The model under review builds one solid part; all positions refer to its coordinate system, in mm. A direction names the side the tool comes from. Give positions to 0.01 mm unless a question says otherwise; leave off trailing zeros. Loops run counter-clockwise (first coordinate to the right, second up) from the corner with the lowest first, then second, coordinate; pieces in that order, holes last. Notation, with made-up numbers: (-36, -13.5) -> (-16, -13.5) arc R17 cw to (-16, 1.5) -> close; hole circle Ø10 at (26, 74.5). An arc over 180 degrees is marked (long way). Write each question's results on one line, items separated by ' | '. Start each with the question number.
Q1. Mouldability with a two-part tool opening along Y and no side actions: class faces 1 (the face through (197, 4, 0)), 2 (the face through (197, 0, 19)), 3 (the face through (390, -4.5, 2.7)) as released by +Y, released by -Y, zero draft, split by the parting line, or undercut.
Q2. We need section C-C (z = -1.5). Write out the cut boundary in (x, y).
Q3. We need section B-B (x = 272). Write out the cut boundary in (y, z).
Q4. Machinability: for faces 4 (the face through (197, 0, -17.5)), 5 (the face through (197, 0, -19)), which of the approach directions +Z, -Z, +X, -X, +Y, -Y give a long, thin tool a straight path to every point of the face, cutting with its end or side? Answer none if there is none.
Q5. We need section A-A (y = 0.5). Write out the cut boundary in (x, z).
Q6. Wall thickness on L1, parallel to Z at x = 326, y = -2.25; L2, parallel to Y at x = 21, z = -13; L3, parallel to X at y = 4.5, z = 8.5: over which ranges is each line inside the solid? List them lowest first. Write a range as [from, to].
from build123d import *

# Parameters (mm, degrees)
SKETCH1_W               = 38
SKETCH1_H               = 11
SKETCH1_W_2             = 35
SKETCH1_H_2             = 8
BOSS_EXTRUDE1_DEPTH     = 400
CUT_EXTRUDE1_DEPTH      = 1
CUT_EXTRUDE1_DEPTH_BACK = 39
CUT_EXTRUDE3_DEPTH      = 1
CUT_EXTRUDE3_DEPTH_BACK = 39


with BuildPart() as part:
    # Sketch1 → Boss-Extrude1 (new body)
    with BuildSketch(Plane(origin=(0, 0, 0), x_dir=(0, 0, -1), z_dir=(1, 0, 0))):
        Rectangle(SKETCH1_W, SKETCH1_H)
        Rectangle(SKETCH1_W_2, SKETCH1_H_2, mode=Mode.SUBTRACT)
    extrude(amount=BOSS_EXTRUDE1_DEPTH)

    # Sketch2 → Cut-Extrude1 (cut, two sides)
    with BuildSketch(Plane(origin=(0, 0, -19), x_dir=(-1, 0, 0), z_dir=(0, 0, -1))) as cut_extrude1_sk:
        Polygon((572.970352137, 578.470352137), (0, 5.5), (-11, -5.5), (-583.970352137, -578.470352137), (561.970352137, -1724.411056412), (1718.911056412, -567.470352137), align=None)
    extrude(amount=CUT_EXTRUDE1_DEPTH, mode=Mode.SUBTRACT)
    extrude(cut_extrude1_sk.sketch, amount=-CUT_EXTRUDE1_DEPTH_BACK, mode=Mode.SUBTRACT)

    # Sketch3 → Cut-Extrude3 (cut, two sides)
    with BuildSketch(Plane(origin=(0, 0, -19), x_dir=(-1, 0, 0), z_dir=(0, 0, -1))) as cut_extrude3_sk:
        Polygon((-972.970352137, 578.470352137), (-400, 5.5), (-389, -5.5), (183.970352137, -578.470352137), (-961.970352137, -1724.411056412), (-2118.911056412, -567.470352137), align=None)
    extrude(amount=CUT_EXTRUDE3_DEPTH, mode=Mode.SUBTRACT)
    extrude(cut_extrude3_sk.sketch, amount=-CUT_EXTRUDE3_DEPTH_BACK, mode=Mode.SUBTRACT)


solid = part.part
Output:
1) face 1: undercut | face 2: zero draft | face 3: released by -Y
2) outline: (0, 5.5) -> (1.5, 4) -> (398.5, 4) -> (400, 5.5) -> close; (9.5, -4) -> (11, -5.5) -> (389, -5.5) -> (390.5, -4) -> close
3) outline: (-5.5, -19) -> (5.5, -19) -> (5.5, 19) -> (-5.5, 19) -> close; hole (-4, -17.5) -> (4, -17.5) -> (4, 17.5) -> (-4, 17.5) -> close
4) face 4: +X, -X | face 5: -Z, +X, -X, +Y, -Y
5) outline: (5, -19) -> (395, -19) -> (395, -17.5) -> (5, -17.5) -> close; (5, 17.5) -> (395, 17.5) -> (395, 19) -> (5, 19) -> close
6) L1: [-19, -17.5], [17.5, 19] | L2: [-5.5, -4], [4, 5.5] | L3: [1, 399]
